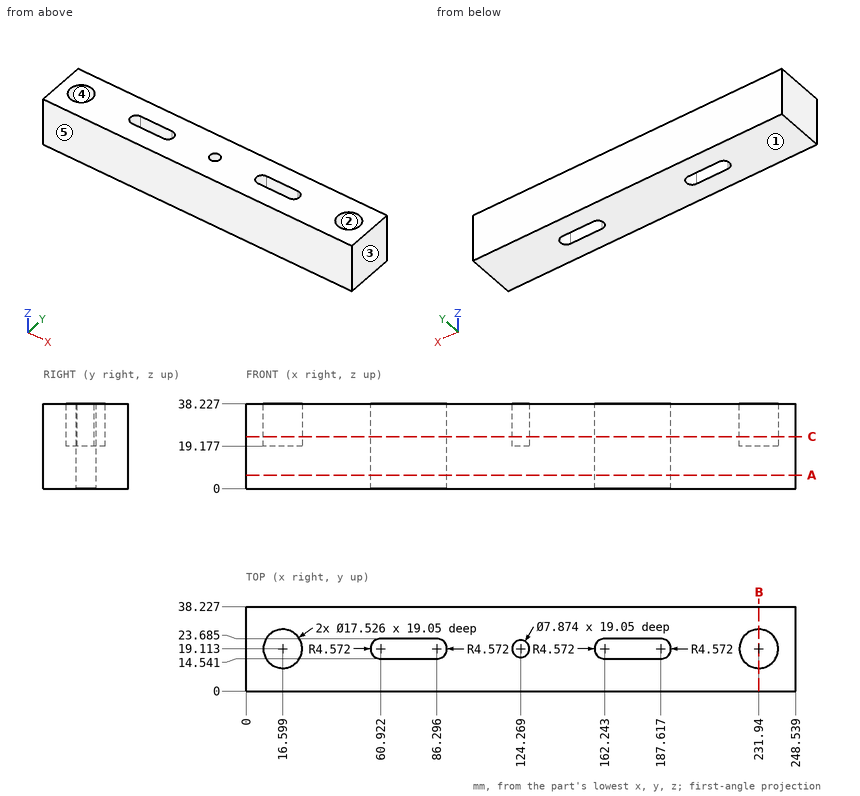
Check sheet for the drawn part. Datum: minimum x, y, z corner. Units: mm. A direction names the side the tool comes from. Coordinates: 2 decimals unless noted, no trailing zeros. Loops run counter-clockwise (first coordinate to the right, second up) from the corner with the lowest first, then second, coordinate; pieces in that order, holes last. Notation, with made-up numbers: M 89,78 L 96,78 A32 ccw 96,115 Z; hole C -26,33.5 d7. An arc over 180 degrees is marked long. Answer as a JSON object with one key per item and string values.
1. Scan lines: L1, parallel to Y at x = 70, z = 35 (1 decimal); L2, parallel to X at y = 27, z = 27.5 (1 decimal); L3, parallel to X at y = 17.5, z = 33.5 (1 decimal). Record each from-to range of solid material in increasing order. Write a range as from..to.
Outcome:
{"L1": "0..14.5, 23.7..38.2", "L2": "0..12.8, 20.4..228.1, 235.8..248.5", "L3": "0..8, 25.2..56.6, 90.6..120.7, 127.9..158, 191.9..223.3, 240.6..248.5"}
2. Sectioned sample at C-C on z = 23.5. Record the cut outline in (x, y) (1 decimal).
Outcome:
{"outline": "M 0,0 L 248.5,0 L 248.5,38.2 L 0,38.2 Z; hole C 16.6,19.1 d17.5; hole M 60.9,14.5 L 86.3,14.5 A4.6 ccw 86.3,23.7 L 60.9,23.7 A4.6 ccw Z; hole C 124.3,19.1 d7.9; hole M 162.2,14.5 L 187.6,14.5 A4.6 ccw 187.6,23.7 L 162.2,23.7 A4.6 ccw Z; hole C 231.9,19.1 d17.5"}
3. Depth check by flat-ended pin: P1, Ø16, axis at x = 231.94, y = 19.11, coming from the +Z side. Enter the tip coordinate at first touch or a pass-through.
Outcome:
{"P1": "z = 19.18"}
4. Release check for a two-part mould opening along X. For the marked faces 3, 4 and 5 record: pulls with the +X half, pulls with the -X half, needs draft (parallel to the pull), parting line crosses it, or undercut.
Outcome:
{"face 3": "pulls with the +X half", "face 4": "undercut", "face 5": "needs draft"}
5. Sectioned sample at A-A on z = 6. Record the cut outline in (x, y) (1 decimal).
Outcome:
{"outline": "M 0,0 L 248.5,0 L 248.5,38.2 L 0,38.2 Z; hole M 60.9,14.5 L 86.3,14.5 A4.6 ccw 86.3,23.7 L 60.9,23.7 A4.6 ccw Z; hole M 162.2,14.5 L 187.6,14.5 A4.6 ccw 187.6,23.7 L 162.2,23.7 A4.6 ccw Z"}
6. Access from +Z, -Z, +X, -X, +Y, -Y to the whole of each face (thin tool, end or side, straight path). Record for the marked faces 1 and 2.
Outcome:
{"face 1": "-Z, +X, -X, +Y, -Y", "face 2": "+Z"}
7. Sectioned sample at B-B on x = 232. Record the cut outline in (y, z), and give its area (3 significant figures).
Outcome:
{"outline": "M 0,0 L 38.23,0 L 38.23,38.23 L 27.88,38.23 L 27.88,19.18 L 10.35,19.18 L 10.35,38.23 L 0,38.23 Z", "area": "1,130 mm²"}
